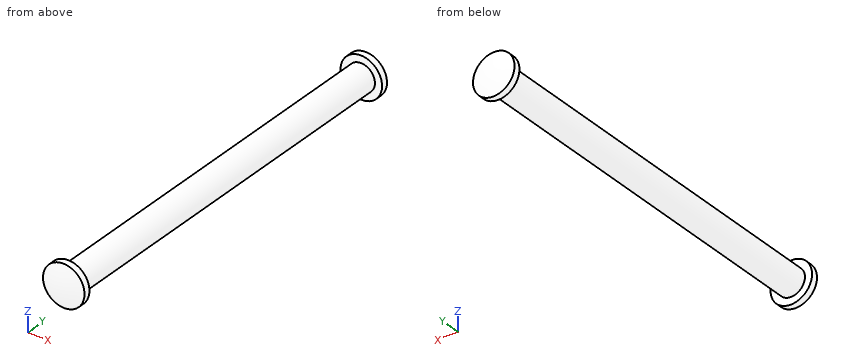
```python
from build123d import *


with BuildPart() as part:
    # Sketch1 → Revolve1 (revolve)
    with BuildSketch(Plane.XY, mode=Mode.PRIVATE) as revolve1_sk:
        with BuildLine():
            Line((0, -19.812), (0, 19.812))
            ThreePointArc((0, 19.812), (1.029625208, 19.727969353), (2.032, 19.478101395))
            Line((2.032, 19.478101395), (2.032, 18.843101395))
            Line((2.032, 18.843101395), (1.3335, 18.843101395))
            Line((1.3335, 18.843101395), (1.3335, -18.843101395))
            Line((1.3335, -18.843101395), (2.032, -18.843101395))
            Line((2.032, -18.843101395), (2.032, -19.478101395))
            ThreePointArc((2.032, -19.478101395), (1.029625208, -19.727969353), (0, -19.812))
        make_face()
    revolve(revolve1_sk.sketch.rotate(Axis((0, -19.812, 0), (0, 1, 0)), 90), axis=Axis((0, -19.812, 0), (0, 1, 0)))


solid = part.part
```
Check sheet for the modelled part. Datum: model origin and axes. Units: mm. Round coordinates to 2 decimals unless told otherwise and drop trailing zeros. Loops run counter-clockwise (first coordinate to the right, second up) from the corner with the lowest first, then second, coordinate; pieces in that order, holes last. Notation, with made-up numbers: (-14.5, 85.25) -> (8.5, 85.25) arc R15 cw to (8.5, 98.25) -> close; hole circle Ø6 at (69, 41). An arc over 180 degrees is marked (long way). Answer in a Markdown table with one row per item.
Q1. Sectioned sample at B-B on x = 0. Enter the section's corners in (y, z).
Data:
| item | result |
|---|---|
| outline | (-19.48, -2.03) -> (-18.84, -2.03) -> (-18.84, -1.33) -> (18.84, -1.33) -> (18.84, -2.03) -> (19.48, -2.03) arc R6.35 ccw to (19.48, 2.03) -> (18.84, 2.03) -> (18.84, 1.33) -> (-18.84, 1.33) -> (-18.84, 2.03) -> (-19.48, 2.03) arc R6.35 ccw to start |
Q2. Sectioned sample at A-A on z = 0. Enter the section's corners in (x, y).
Data:
| item | result |
|---|---|
| outline | (-2.03, -19.48) arc R6.35 ccw to (2.03, -19.48) -> (2.03, -18.84) -> (1.33, -18.84) -> (1.33, 18.84) -> (2.03, 18.84) -> (2.03, 19.48) arc R6.35 ccw to (-2.03, 19.48) -> (-2.03, 18.84) -> (-1.33, 18.84) -> (-1.33, -18.84) -> (-2.03, -18.84) -> close |
Q3. Go/stop test with flat-tipped pins: P1, Ø1, axis at x = 0.5, y = -10, coming from the -Z side; P2, Ø1, axis at x = 1.5, y = -15, coming from the +Z side; P3, Ø1, axis at x = 1.5, z = 0, coming from the +Y side. Record where each tip stops, or that it passes through.
Data:
| item | result |
|---|---|
| P1 | stops at z = -1.33 |
| P2 | stops at z = 0.88 |
| P3 | stops at y = 19.73 |
Q4. Thickness scan on L1, parallel to X at y = -13, z = 0.1; L2, parallel to Y at x = -1.5, z = 0.4; L3, parallel to Y at x = 0, z = 0.15. Record the ranges inside material, lowest first.
Data:
| item | result |
|---|---|
| L1 | x = -1.33 to 1.33 |
| L2 | y = -19.62 to -18.84, 18.84 to 19.62 |
| L3 | y = -19.81 to 19.81 |
Q5. Sectioned sample at C-C on y = -13.5. Enter the section's corners in (x, z), then the cut area to 3 significant figures.
Data:
| item | result |
|---|---|
| outline | circle Ø2.67 at (0, 0) |
| area | 5.59 mm^2 |
